Geometry check sheet. Reference: the model listing, model coordinates, mm. A direction names the side the tool comes from. Coordinates: 2 decimals unless noted, no trailing zeros. Loops run counter-clockwise (first coordinate to the right, second up) from the corner with the lowest first, then second, coordinate; pieces in that order, holes last.
from build123d import *

# Parameters (mm, degrees)
F0_R     = 36
F0_R_2   = 30
F1_DEPTH = 30
F4_DEPTH = 25
F5_DEPTH = 19
F6_DEPTH = 19
F7_DEPTH = 6


with BuildPart() as f1:
    # F0 (on Top) → F1 (new body)
    with BuildSketch(Plane.XY):
        Circle(F0_R)
        Circle(F0_R_2, mode=Mode.SUBTRACT)
    extrude(amount=F1_DEPTH)

    # F3 (on offset) → F4 (join)
    with BuildSketch(Plane.XY.offset(30)):
        with BuildLine():
            Line((0, -36), (0, -30))
            ThreePointArc((0, -30), (-21.213203, -21.213203), (-30, 0))
            ThreePointArc((-30, 0), (-29.994024, 0.598773), (-29.976098, 1.197308))
            Line((-29.976098, 1.197308), (-50.835455, 49))
            Line((-50.835455, 49), (0, 49))
            Line((0, 49), (0, 55))
            Line((0, 55), (-60, 55))
            Line((-60, 55), (-36, 0))
            Line((-36, 0), (-23.334524, -23.334524))
            Line((-23.334524, -23.334524), (0, -36))
        make_face()
        with BuildLine():
            ThreePointArc((30, 0), (21.213203, -21.213203), (0, -30))
            Line((0, -30), (0, -36))
            Line((0, -36), (23.334524, -23.334524))
            Line((23.334524, -23.334524), (36, 0))
            Line((36, 0), (60, 55))
            Line((60, 55), (0, 55))
            Line((0, 55), (0, 49))
            Line((0, 49), (50.835455, 49))
            Line((50.835455, 49), (29.976098, 1.197308))
            ThreePointArc((29.976098, 1.197308), (29.994024, 0.598773), (30, 0))
        make_face()
        with BuildLine():
            ThreePointArc((-29.976098, 1.197308), (-20.785581, 21.632374), (0, 30))
            Line((0, 30), (0, 49))
            Line((0, 49), (-50.835455, 49))
            Line((-50.835455, 49), (-29.976098, 1.197308))
        make_face()
        with BuildLine():
            Line((0, 49), (0, 30))
            ThreePointArc((0, 30), (20.785581, 21.632374), (29.976098, 1.197308))
            Line((29.976098, 1.197308), (50.835455, 49))
            Line((50.835455, 49), (0, 49))
        make_face()
        with BuildLine():
            Line((0, 30), (0, 0))
            Line((0, 0), (0, -30))
            Line((0, -30), (29.453636, 0))
            Line((29.453636, 0), (29.976098, 1.197308))
            ThreePointArc((29.976098, 1.197308), (20.785581, 21.632374), (0, 30))
        make_face()
        with BuildLine():
            Line((0, -30), (0, 0))
            Line((0, 0), (0, 30))
            ThreePointArc((0, 30), (-20.785581, 21.632374), (-29.976098, 1.197308))
            Line((-29.976098, 1.197308), (-29.453636, 0))
            Line((-29.453636, 0), (0, -30))
        make_face()
        with BuildLine():
            ThreePointArc((-30, 0), (-21.213203, -21.213203), (0, -30))
            Line((0, -30), (-29.453636, 0))
            Line((-29.453636, 0), (-30, 0))
        make_face()
        with BuildLine():
            Line((29.453636, 0), (0, -30))
            ThreePointArc((0, -30), (21.213203, -21.213203), (30, 0))
            ThreePointArc((30, 0), (29.994024, 0.598773), (29.976098, 1.197308))
            Line((29.976098, 1.197308), (29.453636, 0))
        make_face()
    extrude(amount=F4_DEPTH)

    # F3 (on offset) → F5 (cut)
    with BuildSketch(Plane.XY.offset(30)):
        with BuildLine():
            ThreePointArc((-30, 0), (-21.213203, -21.213203), (0, -30))
            Line((0, -30), (-29.453636, 0))
            Line((-29.453636, 0), (-30, 0))
        make_face()
        with BuildLine():
            Line((0, -30), (0, 0))
            Line((0, 0), (0, 30))
            ThreePointArc((0, 30), (-20.785581, 21.632374), (-29.976098, 1.197308))
            Line((-29.976098, 1.197308), (-29.453636, 0))
            Line((-29.453636, 0), (0, -30))
        make_face()
        with BuildLine():
            Line((0, 30), (0, 0))
            Line((0, 0), (0, -30))
            Line((0, -30), (29.453636, 0))
            Line((29.453636, 0), (29.976098, 1.197308))
            ThreePointArc((29.976098, 1.197308), (20.785581, 21.632374), (0, 30))
        make_face()
        with BuildLine():
            Line((29.453636, 0), (0, -30))
            ThreePointArc((0, -30), (21.213203, -21.213203), (30, 0))
            ThreePointArc((30, 0), (29.994024, 0.598773), (29.976098, 1.197308))
            Line((29.976098, 1.197308), (29.453636, 0))
        make_face()
    extrude(amount=F5_DEPTH, mode=Mode.SUBTRACT)

    # F3 (on offset) → F6 (cut)
    with BuildSketch(Plane.XY.offset(30)):
        with BuildLine():
            ThreePointArc((-29.976098, 1.197308), (-20.785581, 21.632374), (0, 30))
            Line((0, 30), (0, 49))
            Line((0, 49), (-50.835455, 49))
            Line((-50.835455, 49), (-29.976098, 1.197308))
        make_face()
        with BuildLine():
            Line((0, 49), (0, 30))
            ThreePointArc((0, 30), (20.785581, 21.632374), (29.976098, 1.197308))
            Line((29.976098, 1.197308), (50.835455, 49))
            Line((50.835455, 49), (0, 49))
        make_face()
    extrude(amount=F6_DEPTH, mode=Mode.SUBTRACT)

    # F3 (on offset) → F7 (join)
    with BuildSketch(Plane.XY.offset(30)):
        with BuildLine():
            Line((0, 49), (0, 30))
            ThreePointArc((0, 30), (20.785581, 21.632374), (29.976098, 1.197308))
            Line((29.976098, 1.197308), (50.835455, 49))
            Line((50.835455, 49), (0, 49))
        make_face()
        with BuildLine():
            ThreePointArc((-29.976098, 1.197308), (-20.785581, 21.632374), (0, 30))
            Line((0, 30), (0, 49))
            Line((0, 49), (-50.835455, 49))
            Line((-50.835455, 49), (-29.976098, 1.197308))
        make_face()
    extrude(amount=F7_DEPTH)


solid = f1.part
1) Material ranges on probe 1 along Y at (x, z) = (0, 8.75); probe 2 along Z at (x, y) = (-37, 44), recorded low to high.
Data:
probe 1: y = -36 to -30, 30 to 36
probe 2: z = 30 to 36, 49 to 55
2) Mould release check, pull along Y, two halves, no side actions. Record for faces 1 (the cylindrical face through (-4.686, 35.694, 14.79)), 2 (the flat face through (40.26, 24.76, 42.41)), 3 (the flat face through (29.58, -11.83, 42.32)), 4 (the flat face through (-1, 40, 30)): +Y half, -Y half, draft (parallel to the pull), parting line (faces both ways), or undercut.
Data:
face 1: parting line
face 2: undercut
face 3: -Y half
face 4: draft
3) Section check B-B on x = -46.5. Record the cut outline in (y, z).
Data:
outline: (24.06, 30) - (55, 30) - (55, 55) - (24.06, 55) - close; hole (39.06, 36) - (49, 36) - (49, 49) - (39.06, 49) - close
4) Depth check by flat-ended pin: pin 1 (10.5 mm diameter, centred on x = -5.5, z = 40.5, fed in from -Y); pin 2 (10 mm diameter, centred on x = 44, z = 5.5, fed in from -Y); pin 3 (1 mm diameter, centred on y = 9.5, z = 9.5, fed in from -X); pin 4 (2 mm diameter, centred on x = -36, z = 40, fed in from -Y). Enter the tip coordinate at first touch or a pass-through.
Data:
pin 1: stops at y = -35.86
pin 2: passes through
pin 3: stops at x = -34.86
pin 4: stops at y = -1.84
5) Section check D-D on x = -26.5. Record the cut outline in (y, z).
Data:
outline: (-24.37, 0) - (-14.06, 0) - (-14.06, 49) - (49, 49) - (49, 36) - (14.06, 36) - (14.06, 0) - (24.37, 0) - (24.37, 30) - (55, 30) - (55, 55) - (-17.5, 55) - (-17.5, 30) - (-24.37, 30) - close
6) Access from +Z, -Z, +X, -X, +Y, -Y to the whole of each face (thin tool, end or side, straight path). Record for faces 5 (the flat face through (-11.83, -29.58, 42.32)), 6 (the flat face through (23, -25, 30)), 7 (the flat face through (-14, 27, 0)), 8 (the flat face through (-1, 19, 49)).
Data:
face 5: +Z, -X, -Y
face 6: +Z, +X, -Y
face 7: -Z, +X, -X, +Y, -Y
face 8: none
7) Section check C-C on z = 47. Record the cut outline in (x, y).
Data:
outline: (-60, 55) - (-36, 0) - (-23.33, -23.33) - (0, -36) - (23.33, -23.33) - (36, 0) - (60, 55) - close; hole (-50.84, 49) - (-29.98, 1.2) arc R30 ccw to (-30, 0) arc R30 ccw to (0, -30) arc R30 ccw to (30, 0) arc R30 ccw to (29.98, 1.2) - (50.84, 49) - close
8) Section check A-A on z = 32. Record the cut outline in (x, y), and give its area (3 significant figures).
Data:
outline: (-60, 55) - (-36, 0) - (-23.33, -23.33) - (0, -36) - (23.33, -23.33) - (36, 0) - (60, 55) - close; hole (-30, 0) arc R30 ccw to (0, -30) arc R30 ccw to (30, 0) arc R30 ccw to (29.98, 1.2) arc R30 ccw to (0, 30) arc R30 ccw to (-29.98, 1.2) arc R30 ccw to start
area: 4,130 mm2
